Geometry: see drawing. Coordinates: mm, zero at the bounding-box minimum. A direction names the side the tool comes from. Coordinates: 2 decimals unless noted, no trailing zeros. Order: outer loops, then holes, each group sorted by start corner. A loop starts at its lowest first (then second) coordinate and runs counter-clockwise, first axis right, second up. Notation, with made-up numbers: M 33,2 L 85,2 A30 cw 85,40 Z; hole C -28,-4 d9. An arc over 180 degrees is marked long. Answer in a Markdown table with one row per item.
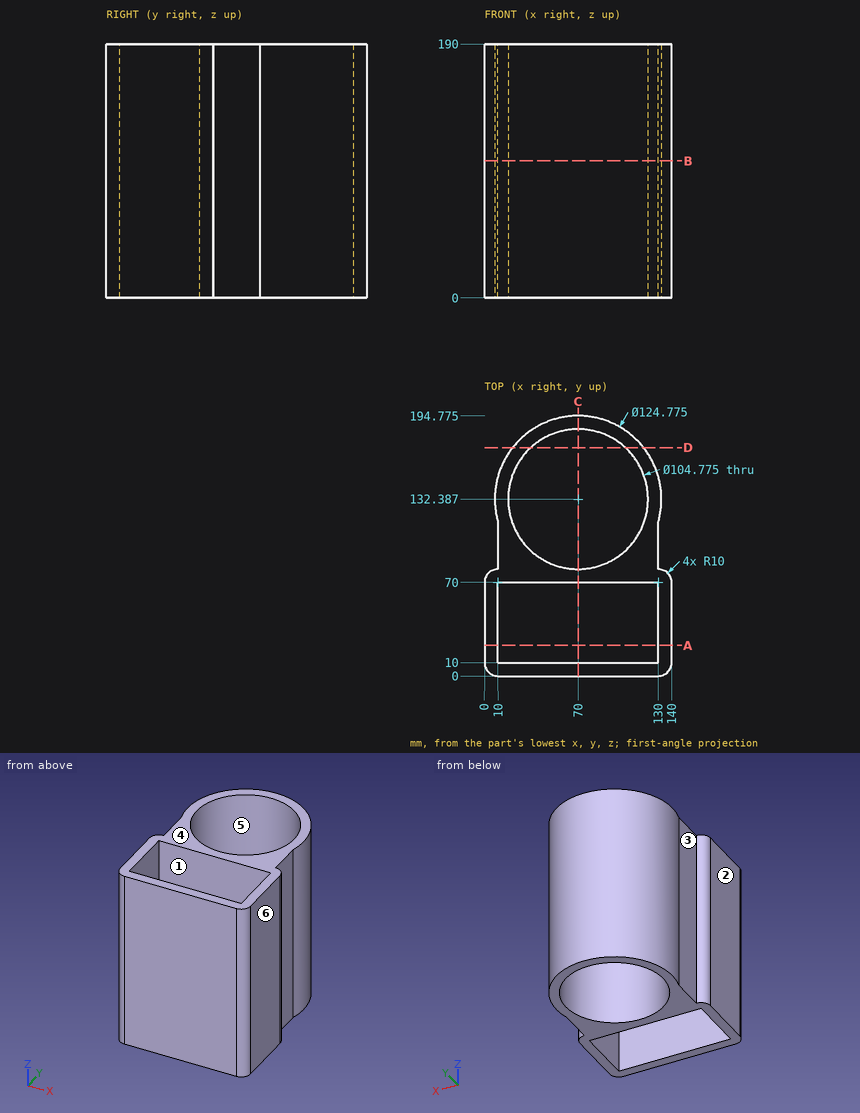
1) Cut plane B-B, the plane z = 102.5. Output: boundary loops of the cut face in (x, y) (1 decimal), and give its area (3 significant figures).
Resolved:
| item | result |
|---|---|
| outline | M 0,10 A10 ccw 10,0 L 130,0 A10 ccw 140,10 L 140,70 A10 ccw 130,80 L 130,115.3 A62.4 ccw long 10,115.3 L 10,80 A10 ccw 0,70 Z; hole M 10,10 L 130,10 L 130,70 L 10,70 Z; hole C 70,132.4 d104.8 |
| area | 7,750 mm2 |
2) Cut plane C-C, the plane x = 70. Output: boundary loops of the cut face in (y, z) (1 decimal), and give its area (3 significant figures).
Resolved:
| item | result |
|---|---|
| outline | M 0,0 L 10,0 L 10,190 L 0,190 Z; M 70,0 L 80,0 L 80,190 L 70,190 Z; M 184.8,0 L 194.8,0 L 194.8,190 L 184.8,190 Z |
| area | 5,700 mm2 |
3) Material intervals for probe 1 along Y at (x, z) = (70.5, 121); probe 2 along X at (y, z) = (30, 146); probe 3 along Y at (x, z) = (86, 135), sorted ascending.
Resolved:
| item | result |
|---|---|
| probe 1 | y = 0 to 10, 70 to 80, 184.77 to 194.77 |
| probe 2 | x = 0 to 10, 130 to 140 |
| probe 3 | y = 0 to 10, 70 to 82.5, 182.27 to 192.69 |
4) Reachability of the marked faces 1, 2 and 3 from +Z, -Z, +X, -X, +Y, -Y: full face, straight path, thin tool, end or side. Return the list, or none.
Resolved:
| item | result |
|---|---|
| face 1 | +Z, -Z |
| face 2 | +Z, -Z, -X, +Y, -Y |
| face 3 | +Z, -Z, -X |
5) Cut plane A-A, the plane y = 23. Output: boundary loops of the cut face in (x, z).
Resolved:
| item | result |
|---|---|
| outline | M 0,0 L 10,0 L 10,190 L 0,190 Z; M 130,0 L 140,0 L 140,190 L 130,190 Z |
6) Mould query, pull axis X, two halves, no side actions, for the marked faces 4, 5 and 6. Classes: +X half, -X half, draft (parallel to the pull), parting line (faces both ways), or undercut.
Resolved:
| item | result |
|---|---|
| face 4 | draft |
| face 5 | undercut |
| face 6 | +X half |
7) Cut plane D-D, the plane y = 171. Output: boundary loops of the cut face in (x, z) (1 decimal), and give its area (3 significant figures).
Resolved:
| item | result |
|---|---|
| outline | M 21,0 L 34.6,0 L 34.6,190 L 21,190 Z; M 105.4,0 L 119,0 L 119,190 L 105.4,190 Z |
| area | 5,170 mm2 |
8) Contact query for flat-ended pins moving along their axis: pin 1 (4 mm diameter, centred on y = 79.5, z = 150, fed in from -X) (1 decimal); pin 2 (3 mm diameter, centred on y = 157, z = 112, fed in from +X); pin 3 (1 mm diameter, centred on y = 110.5, z = 159.5, fed in from +X). Output: stop coordinate, or through.
Resolved:
| item | result |
|---|---|
| pin 1 | stops at x = 3.4 |
| pin 2 | stops at x = 127.95 |
| pin 3 | stops at x = 130 |
